Job drawing, mm, ordinate dimensions from the low corner. One solid piece. A direction names the side the tool comes from. Coordinates: 2 decimals unless noted, no trailing zeros. Loops run counter-clockwise (first coordinate to the right, second up) from the corner with the lowest first, then second, coordinate; pieces in that order, holes last. Notation, with made-up numbers: (-2, -38.5) -> (27, -38.5) arc R15 ccw to (27, -31.5) -> close; hole circle Ø10 at (83, 72). An arc over 180 degrees is marked (long way). Use one line per item in the form item = value. Start each with the question number.
(1) Drill centre lines: L1, parallel to X at y = 10.5, z = 2.6; L2, parallel to Y at x = 6.25, z = 0.3; L3, parallel to Y at x = 1, z = 0.75. Where is each one in solid material? Low to high. Write a range as [from, to].
(2) Band-saw the part on A-A on y = 11. Give the cut face in (x, z), then the cut area to 3 significant figures.
(3) Band-saw the part on C-C on x = 7.25. Give the cut face in (y, z).
(4) 3-axis set-ups, long thin cutter, end or side, ignore diameter. For the marked faces 5 and 6: which of +Z, -Z, +X, -X, +Y, -Y reach the whole face in a straight line?
(5) Band-saw the part on D-D on y = 1. Give the cut face in (x, z), then the cut area to 3 significant figures.
(6) Mould opens along X. For the marked faces 1, 2, 3 and 4 say: +X half, -X half, draft (parallel to the pull), parting line (faces both ways), or undercut.
(7) Band-saw the part on B-B on z = 2.35. Give the cut face in (x, y).
(8) Pin check, flat tip, straight feed: P1, Ø0.9, axis at x = 8.5, z = 2, coming from the +Y side. Stop position of the tip, or through.
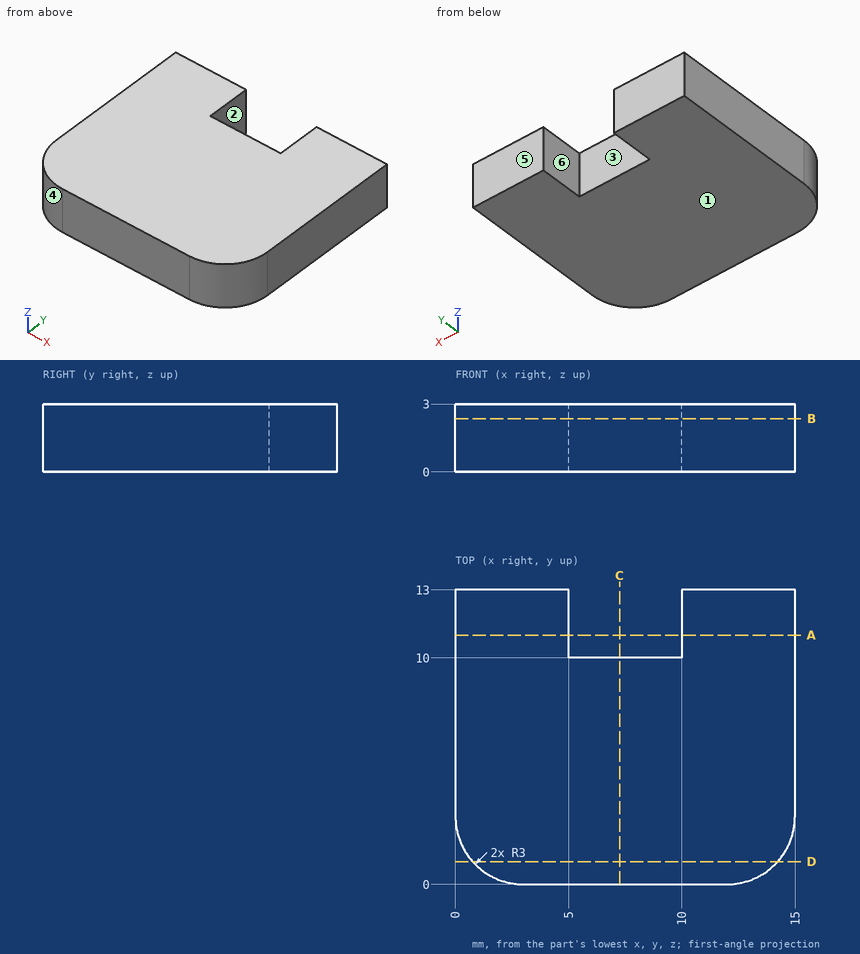
A:
q1.L1 = [0, 5], [10, 15]
q1.L2 = [0, 10]
q1.L3 = [0.76, 13]
q2.outline = (0, 0) -> (5, 0) -> (5, 3) -> (0, 3) -> close; (10, 0) -> (15, 0) -> (15, 3) -> (10, 3) -> close
q2.area = 30.0 mm²
q3.outline = (0, 0) -> (10, 0) -> (10, 3) -> (0, 3) -> close
q4.face_5 = +Z, -Z, +X, -X, +Y
q4.face_6 = +Z, -Z, +Y
q5.outline = (0.76, 0) -> (14.24, 0) -> (14.24, 3) -> (0.76, 3) -> close
q5.area = 40.4 mm²
q6.face_1 = draft
q6.face_2 = undercut
q6.face_3 = undercut
q6.face_4 = -X half
q7.outline = (0, 3) arc R3 ccw to (3, 0) -> (12, 0) arc R3 ccw to (15, 3) -> (15, 13) -> (10, 13) -> (10, 10) -> (5, 10) -> (5, 13) -> (0, 13) -> close
q8.P1 = 10
